Can you work these out from the model? Positions are in its coordinate system, mm. A direction names the side the tool comes from. Coordinates: 2 decimals unless noted, no trailing zeros. Order: outer loops, then holes, each group sorted by start corner. A loop starts at its lowest first (then second) coordinate and runs counter-clockwise, first axis right, second up. Notation, with made-up numbers: (-27, -31.75) -> (-18, -31.75) arc R25 ccw to (-18, 7.25) -> close; hole circle Ø6 at (15.5, -21.5). An arc over 180 degrees is marked (long way). Return JSON: item names as keys, results as strings. Group by question number.
1) For pin 1 (4 mm diameter, centred on x = 57, z = -150, fed in from -Y); pin 2 (6 mm diameter, centred on y = 31, z = -136.5, fed in from +X), each with a flat end and sliding along its axis, tell me the tip position at first contact or that it passes through.
2) Thinking about a two-plate mould opening in Y: for faces 4 (the flat face through (54, 109, -91)), 5 (the flat face through (102, -6, -175)), 6 (the flat face through (54, 52, 3)), 7 (the flat face through (54, 34, -180)), which applies, +Y half, -Y half, draft (parallel to the pull), parting line (faces both ways), or undercut?
3) For faces 1 (the flat face through (110, -1, -90)), 2 (the flat face through (54, 106, -89)), 3 (the flat face through (54, -3, -91)), which set-ups out of +Z, -Z, +X, -X, +Y, -Y let a thin tool reach every point of the face, with its end or its side?
4) If we section it at B-B, the plane y = 93.5: Please give me the cut outline in (x, z), then the cut area to 3 significant figures.
5) If we section it at C-C, the plane z = -96.5: Please give me the cut outline in (x, y).
6) If we section it at A-A, the plane x = 48: Please give me the cut outline in (y, z), then the cut area to 3 significant figures.
7) If I drill on probe 1 along Y at (x, z) = (54, -22.5); probe 2 along Z at (x, y) = (15.5, 64); probe 3 along Z at (x, y) = (67.5, 88.5), over which ranges is the centre line in solid material (lowest first)? Write a range as from..to.
from build123d import *

# Parameters (mm, degrees)
BOSS_EXTRUDE1_DEPTH           = 110
SKETCH2_W                     = 186
SKETCH2_H                     = 112
BOSS_EXTRUDE2_DEPTH           = 3
SKETCH3_W                     = 16
SKETCH3_H                     = 16
BOSS_EXTRUDE3_DEPTH           = 3
BOSS_EXTRUDE3_DRAFT           = 50
BOSS_EXTRUDE3_PROFILE_2_DEPTH = 3
BOSS_EXTRUDE3_PROFILE_2_DRAFT = 50
BOSS_EXTRUDE3_PROFILE_3_DEPTH = 3
BOSS_EXTRUDE3_PROFILE_3_DRAFT = 50
BOSS_EXTRUDE3_PROFILE_4_DEPTH = 3
BOSS_EXTRUDE3_PROFILE_4_DRAFT = 50


with BuildPart() as part:
    # Sketch1 → Boss-Extrude1 (new body)
    with BuildSketch(Plane(origin=(0, 0, 0), x_dir=(0, 0, -1), z_dir=(1, 0, 0))):
        Polygon((-3, 0), (-3, 106), (-3, 109), (183, 109), (183, 106), (183, 0), (183, -3), (-3, -3), align=None)
        Polygon((0, 0), (0, 6), (3, 25), (3, 31), (0, 31), (0, 37), (3, 61), (3, 67), (0, 67), (0, 106), (180, 106), (180, 67), (177, 67), (177, 61), (180, 37), (180, 31), (177, 31), (177, 25), (180, 6), (180, 0), align=None, mode=Mode.SUBTRACT)
    extrude(amount=BOSS_EXTRUDE1_DEPTH)

    # Sketch2 → Boss-Extrude2 (add)
    with BuildSketch(Plane.ZY):
        with Locations((-90, 53)):
            Rectangle(SKETCH2_W, SKETCH2_H)
    extrude(amount=BOSS_EXTRUDE2_DEPTH)


with BuildPart() as boss_extrude3_tool:
    # Sketch3 → Boss-Extrude3 (with draft: the straight prism first)
    with BuildSketch(Plane.XZ.offset(3)):
        with Locations((5, -5)):
            Rectangle(SKETCH3_W, SKETCH3_H)
    extrude(amount=BOSS_EXTRUDE3_DEPTH)
    # Boss-Extrude3: the draft: its side faces are tilted about the plane it starts from
    boss_extrude3_sides = [boss_extrude3_tool.faces().sort_by_distance(p)[0] for p in [
        (-3, -4.5, -5),
        (5, -4.5, -13),
        (13, -4.5, -5),
        (5, -4.5, 3),
    ]]
    draft(boss_extrude3_sides, Plane.XZ.offset(3), BOSS_EXTRUDE3_DRAFT)


with BuildPart() as part_1:
    add(part.part)

    # Boss-Extrude3: add boss_extrude3_tool
    add(boss_extrude3_tool.part)


with BuildPart() as boss_extrude3_profile_2_tool:
    # Sketch3 → Boss-Extrude3 profile 2 (with draft: the straight prism first)
    with BuildSketch(Plane.XZ.offset(3)):
        with Locations((102, -5)):
            Rectangle(SKETCH3_W, SKETCH3_H)
    extrude(amount=BOSS_EXTRUDE3_PROFILE_2_DEPTH)
    # Boss-Extrude3 profile 2: the draft: its side faces are tilted about the plane it starts from
    boss_extrude3_profile_2_sides = [boss_extrude3_profile_2_tool.faces().sort_by_distance(p)[0] for p in [
        (102, -4.5, 3),
        (94, -4.5, -5),
        (102, -4.5, -13),
        (110, -4.5, -5),
    ]]
    draft(boss_extrude3_profile_2_sides, Plane.XZ.offset(3), BOSS_EXTRUDE3_PROFILE_2_DRAFT)


with BuildPart() as part_2:
    add(part_1.part)

    # Boss-Extrude3 profile 2: add boss_extrude3_profile_2_tool
    add(boss_extrude3_profile_2_tool.part)


with BuildPart() as boss_extrude3_profile_3_tool:
    # Sketch3 → Boss-Extrude3 profile 3 (with draft: the straight prism first)
    with BuildSketch(Plane.XZ.offset(3)):
        with Locations((102, -175)):
            Rectangle(SKETCH3_W, SKETCH3_H)
    extrude(amount=BOSS_EXTRUDE3_PROFILE_3_DEPTH)
    # Boss-Extrude3 profile 3: the draft: its side faces are tilted about the plane it starts from
    boss_extrude3_profile_3_sides = [boss_extrude3_profile_3_tool.faces().sort_by_distance(p)[0] for p in [
        (110, -4.5, -175),
        (102, -4.5, -167),
        (94, -4.5, -175),
        (102, -4.5, -183),
    ]]
    draft(boss_extrude3_profile_3_sides, Plane.XZ.offset(3), BOSS_EXTRUDE3_PROFILE_3_DRAFT)


with BuildPart() as part_3:
    add(part_2.part)

    # Boss-Extrude3 profile 3: add boss_extrude3_profile_3_tool
    add(boss_extrude3_profile_3_tool.part)


with BuildPart() as boss_extrude3_profile_4_tool:
    # Sketch3 → Boss-Extrude3 profile 4 (with draft: the straight prism first)
    with BuildSketch(Plane.XZ.offset(3)):
        with Locations((5, -175)):
            Rectangle(SKETCH3_W, SKETCH3_H)
    extrude(amount=BOSS_EXTRUDE3_PROFILE_4_DEPTH)
    # Boss-Extrude3 profile 4: the draft: its side faces are tilted about the plane it starts from
    boss_extrude3_profile_4_sides = [boss_extrude3_profile_4_tool.faces().sort_by_distance(p)[0] for p in [
        (5, -4.5, -183),
        (13, -4.5, -175),
        (5, -4.5, -167),
        (-3, -4.5, -175),
    ]]
    draft(boss_extrude3_profile_4_sides, Plane.XZ.offset(3), BOSS_EXTRUDE3_PROFILE_4_DRAFT)


with BuildPart() as part_4:
    add(part_3.part)

    # Boss-Extrude3 profile 4: add boss_extrude3_profile_4_tool
    add(boss_extrude3_profile_4_tool.part)


solid = part_4.part
Result sheet:
{
 "1": {"pin 1": "stops at y = -3", "pin 2": "stops at x = 0"},
 "2": {"face 4": "+Y half", "face 5": "-Y half", "face 6": "draft", "face 7": "undercut"},
 "3": {"face 1": "+Z, -Z, +X, +Y, -Y", "face 2": "+X", "face 3": "-Y"},
 "4": {"outline": "(-3, -183) -> (110, -183) -> (110, -180) -> (0, -180) -> (0, 0) -> (110, 0) -> (110, 3) -> (-3, 3) -> close", "area": "1,220 mm2"},
 "5": {"outline": "(-3, -3) -> (110, -3) -> (110, 0) -> (0, 0) -> (0, 106) -> (110, 106) -> (110, 109) -> (-3, 109) -> close"},
 "6": {"outline": "(-3, -183) -> (109, -183) -> (109, 3) -> (-3, 3) -> close; hole (0, -180) -> (6, -180) -> (25, -177) -> (31, -177) -> (31, -180) -> (37, -180) -> (61, -177) -> (67, -177) -> (67, -180) -> (106, -180) -> (106, 0) -> (67, 0) -> (67, -3) -> (61, -3) -> (37, 0) -> (31, 0) -> (31, -3) -> (25, -3) -> (6, 0) -> (0, 0) -> close", "area": "1,950 mm2"},
 "7": {"probe 1": "y = -3..0, 106..109", "probe 2": "z = -183..-177, -3..3", "probe 3": "z = -183..-180, 0..3"}
}
